Could you check a few things on this model? Use its own coordinates, in mm. A direction names the side the tool comes from. Coordinates: 2 decimals unless noted, no trailing zeros. Order: outer loops, then holes, each group sorted by start corner. A loop starts at its lowest first (then second) coordinate and runs counter-clockwise, first axis right, second up. Notation, with made-up numbers: M 20,29.5 L 66,29.5 A19 ccw 66,36.5 Z; hole C 17,-6.5 d10. An arc over 180 degrees is marked long. Put each result on its own line as item: value. Start each with the question number.
Autodesk Inventor part; units mm, degrees
ref_plane "YZ Plane" through (0, 0, 0) normal (1, 0, 0) x (0, 1, 0)
ref_plane "XZ Plane" through (0, 0, 0) normal (0, 1, 0) x (-1, 0, 0)
ref_plane "XY Plane" through (0, 0, 0) normal (0, 0, 1) x (1, 0, 0)
sketch "Sketch1" plane through (0, 0, 0) normal (1, 0, 0) x (0, 1, 0)
  line L0 (15.7193, -14.4333) -> (-9.6807, -14.4333)
  line L1 (-9.6807, -14.4333) -> (-9.6807, 10.9667)
  line L2 (-9.6807, 10.9667) -> (15.7193, 10.9667)
  line L3 (15.7193, 10.9667) -> (15.7193, -14.4333)
  line L4 (15.7193, -14.4333) -> (-9.6807, 10.9667) construction
  line L5 (-9.6807, -14.4333) -> (15.7193, 10.9667) construction
  point P0 (0, 0)
  point P1 (3.0193, -1.7333)
  dimension "d0" = 25.4
  dimension "d1" = 25.4
extrude "Extrusion1" add sketch "Sketch1" along normal blind 25.4
sketch "Sketch2" plane through (0, -9.6807, 10.9667) normal (0, 0, 1) x (1, 0, 0)
  circle A0 centre (12.7, 12.7) radius 2.3749
  point P0 (0, 9.6807)
  dimension "d4" = 4.7498
sketch "Sketch3" plane through (0, -9.6807, 10.9667) normal (0, 0, 1) x (1, 0, 0)
  line L0 (0, 0) -> (0, 25.4)
  line L1 (0, 0) -> (25.4, 0)
  line L2 (25.4, 25.4) -> (25.4, 0)
  line L3 (0, 25.4) -> (25.4, 25.4)
  point P0 (0, 9.6807)
extrude "Extrusion2" cut sketch "Sketch2" against normal blind 1.27
sketch "Sketch4" plane through (0, 15.7193, 10.9667) normal (0, 1, 0) x (1, 0, 0)
  circle A0 centre (6.3453, 19.0547) radius 2.3749
  circle A1 centre (12.7, 12.7) radius 2.3749
  circle A2 centre (19.0547, 6.3453) radius 2.3749
  point P0 (0, 10.9667)
  dimension "d7" = 4.7498
  dimension "d8" = 4.7498
  dimension "d9" = 4.7498
extrude "Extrusion3" cut sketch "Sketch4" against normal blind 1.27
sketch "Sketch5" plane through (0, -9.6807, -14.4333) normal (0, -1, 0) x (1, 0, 0)
  circle A0 centre (6.3453, 19.0547) radius 2.3749
  circle A1 centre (19.0547, 19.0547) radius 2.3749
  circle A2 centre (6.3453, 6.3453) radius 2.3749
  circle A3 centre (19.0547, 6.3453) radius 2.3749
  point P0 (0, 14.4333)
  dimension "d12" = 4.7498
  dimension "d13" = 4.7498
  dimension "d14" = 4.7498
  dimension "d15" = 4.7498
extrude "Extrusion4" cut sketch "Sketch5" against normal blind 1.27
sketch "Sketch6" plane through (0, -9.6807, -14.4333) normal (0, 0, -1) x (-1, 0, 0)
  circle A0 centre (-19.0556, 19.0556) radius 2.3749
  circle A1 centre (-6.3444, 19.0556) radius 2.3749
  circle A2 centre (-6.3444, 6.3444) radius 2.3749
  circle A3 centre (-19.0556, 6.3444) radius 2.3749
  circle A4 centre (-6.3444, 12.7) radius 2.3749
  circle A5 centre (-19.0556, 12.7) radius 2.3749
  point P0 (0, 9.6807)
  dimension "d18" = 4.7498
  dimension "d19" = 4.7498
  dimension "d20" = 4.7498
  dimension "d21" = 4.7498
  dimension "d22" = 4.7498
  dimension "d23" = 4.7498
extrude "Extrusion5" cut sketch "Sketch6" against normal blind 1.27
sketch "Sketch7" plane through (0, 0, 0) normal (-1, 0, 0) x (0, 0, 1)
  line L0 (-14.4333, 15.7193) -> (-14.4333, -9.6807)
  line L1 (-14.4333, -9.6807) -> (10.9667, -9.6807)
  line L2 (10.9667, -9.6807) -> (10.9667, 15.7193)
  line L3 (10.9667, 15.7193) -> (-14.4333, 15.7193)
  circle A0 centre (-8.0833, 9.3693) radius 2.3749
  circle A1 centre (4.6222, 9.3693) radius 2.3749
  circle A2 centre (4.6222, -3.3307) radius 2.3749
  circle A3 centre (-8.0833, -3.3307) radius 2.3749
  circle A4 centre (-1.7333, 3.0193) radius 2.3749
  point P0 (0, 0)
  dimension "d26" = 6.35
  dimension "d27" = 6.35
  dimension "d28" = 6.35
  dimension "d29" = 6.3444
  dimension "d30" = 6.35
  dimension "d31" = 6.3444
  dimension "d32" = 6.35
  dimension "d33" = 6.35
  dimension "d34" = 12.7
  dimension "d35" = 12.7
  dimension "d36" = 4.7498
  dimension "d37" = 4.7498
  dimension "d38" = 4.7498
  dimension "d39" = 4.7498
  dimension "d40" = 4.7498
extrude "Extrusion6" cut sketch "Sketch7" against normal blind 1.27 contours A0 | A1 | A2 | A3 | A4
sketch "Sketch8" plane through (25.4, 0, 0) normal (1, 0, 0) x (0, 0, -1)
  line L0 (14.4333, -9.6807) -> (14.4333, 15.7193)
  line L1 (14.4333, 15.7193) -> (-10.9667, 15.7193)
  line L2 (-10.9667, 15.7193) -> (-10.9667, -9.6807)
  line L3 (-10.9667, -9.6807) -> (14.4333, -9.6807)
  circle A0 centre (-4.6167, 9.3693) radius 2.3749
  circle A1 centre (8.0833, -3.3307) radius 2.3749
  point P0 (0, 0)
  dimension "d43" = 4.7498
  dimension "d44" = 4.7498
  dimension "d45" = 6.35
  dimension "d46" = 6.35
  dimension "d47" = 6.35
  dimension "d48" = 6.35
extrude "Extrusion7" cut sketch "Sketch8" against normal blind 1.27 contours A0 | A1
Item 1: If we section it at D-D on x = 5.75: Write out the boundary of the cut face in (y, z).
Item 2: For pin 1 Ø4 at (x, y) = (19, -2.5) entering from -Z; pin 2 Ø3 at (x, z) = (19.05, -8.09) entering from -Y; pin 3 Ø3 at (x, z) = (6.35, -8.09) entering from +Y; pin 4 Ø1.4 at (x, y) = (18.5, 8.5) entering from -Z, each with a flat end and sliding along its axis, tell me the tip position at first contact or that it passes through.
Item 3: For faces 4 (the cylindrical face through (20.94, -4.78, -13.81)), 5 (the cylindrical face through (14.894, 15.093, -0.824)), 6 (the cylindrical face through (4.46, -9.05, 3.18)), 7 (the flat face through (1.27, -3, -8)), 8 (the flat face through (13, 3, -14.433)), which set-ups out of +Z, -Z, +X, -X, +Y, -Y let a thin tool reach every point of the face, with its end or its side?
Item 4: I need wall thicknesses on probe 1 along Z at (x, y) = (12.7, 15.25); probe 2 along Z at (x, y) = (4.5, 4.25); probe 3 along X at (y, z) = (9, -9.25). Which ranges of each line are inside material? Lowest first, please.
Item 5: If we section it at A-A on x = 12.7: Write out the boundary of the cut face in (y, z).
Item 6: If we mould it in two halves opening along X, with no side actions, what happens to faces 1 (the flat face through (6, 14.449, -8)), 2 (the flat face through (0, 0, -2)), 3 (the cylindrical face through (0.626, -2.617, -5.818))? For each: released by +X, released by -X, zero draft, split by the parting line, or undercut.
Item 7: If we section it at B-B on z = -9: Write out the boundary of the cut face in (x, y), then the cut area to 3 significant figures.
Item 8: If we section it at C-C on y = -1.5: Write out the boundary of the cut face in (x, z), then the cut area to 3 significant figures.
Geometry check:
1. outline: M -9.68,-14.43 L -5.64,-14.43 L -5.64,-13.16 L -1.04,-13.16 L -1.04,-14.43 L 0.72,-14.43 L 0.72,-13.16 L 5.32,-13.16 L 5.32,-14.43 L 7.08,-14.43 L 7.08,-13.16 L 11.67,-13.16 L 11.67,-14.43 L 15.72,-14.43 L 15.72,-10.39 L 14.45,-10.39 L 14.45,-5.79 L 15.72,-5.79 L 15.72,10.97 L -9.68,10.97 L -9.68,6.92 L -8.41,6.92 L -8.41,2.32 L -9.68,2.32 L -9.68,-5.79 L -8.41,-5.79 L -8.41,-10.39 L -9.68,-10.39 Z
2. pin 1: stops at z = -14.43
2. pin 2: stops at y = -8.41
2. pin 3: stops at y = 14.45
2. pin 4: stops at z = -13.16
3. face 4: -Z
3. face 5: +Y
3. face 6: -Y
3. face 7: -X
3. face 8: -Z, +X, -X, +Y, -Y
4. probe 1: z = -14.43 to -4.11, 0.64 to 10.97
4. probe 2: z = -13.16 to 10.97
4. probe 3: x = 1.27 to 25.4
5. outline: M -9.68,-14.43 L 15.72,-14.43 L 15.72,-4.11 L 14.45,-4.11 L 14.45,0.64 L 15.72,0.64 L 15.72,10.97 L 5.39,10.97 L 5.39,9.7 L 0.64,9.7 L 0.64,10.97 L -9.68,10.97 Z
6. face 1: undercut
6. face 2: released by -X
6. face 3: zero draft
7. outline: M 0,-9.68 L 4.15,-9.68 L 4.15,-8.41 L 8.54,-8.41 L 8.54,-9.68 L 16.86,-9.68 L 16.86,-8.41 L 21.25,-8.41 L 21.25,-9.68 L 25.4,-9.68 L 25.4,-5.52 L 24.13,-5.52 L 24.13,-1.14 L 25.4,-1.14 L 25.4,15.72 L 8.54,15.72 L 8.54,14.45 L 4.15,14.45 L 4.15,15.72 L 0,15.72 L 0,11.56 L 1.27,11.56 L 1.27,7.18 L 0,7.18 L 0,-1.14 L 1.27,-1.14 L 1.27,-5.52 L 0,-5.52 Z
7. area: 612 mm²
8. outline: M 0,-14.43 L 4.84,-14.43 L 4.84,-13.16 L 7.85,-13.16 L 7.85,-14.43 L 17.55,-14.43 L 17.55,-13.16 L 20.56,-13.16 L 20.56,-14.43 L 25.4,-14.43 L 25.4,-9.6 L 24.13,-9.6 L 24.13,-6.57 L 25.4,-6.57 L 25.4,10.97 L 0,10.97 L 0,6.14 L 1.27,6.14 L 1.27,3.11 L 0,3.11 L 0,-6.57 L 1.27,-6.57 L 1.27,-9.6 L 0,-9.6 Z
8. area: 626 mm²
